Part model, mm, in its own coordinate system. A direction names the side the tool comes from. Round coordinates to 2 decimals unless told otherwise and drop trailing zeros. Write each loop counter-clockwise with the first axis right and the second up, starting at its lowest first coordinate (ties: lowest second). Pieces come first, ordered by that corner, then holes.
1) Saw through at D-D on x = -7.5. Write the cut outline in (y, z).
2) Flat gauge pins, fed straight in: pin 1 (14 mm diameter, centred on x = 0, y = 0, fed in from +Z); pin 2 (3 mm diameter, centred on x = 2, y = -10.5, fed in from -Z); pin 3 (4.5 mm diameter, centred on x = -18.415, z = 25.4, fed in from -Y); pin 4 (14 mm diameter, centred on x = -17.5, z = 38, fed in from +Y). Where does each tip first touch, or does it go through?
3) Which spindle directions (+Z, -Z, +X, -X, +Y, -Y) get a long thin tool onto all of the face, cutting with end or side? Do faces 1 (the flat face through (-1, -25.4, 25)), 2 (the flat face through (-1, -22.098, 27)). Say none if no direction does.
4) Saw through at A-A on z = 25.4. Write the cut outline in (x, y), and give its area (3 significant figures).
5) Pull direction Z, two halves, no side cores. Call faces 3 (the flat face through (-1, 7, 3.302)), 4 (the cylindrical face through (-16.01, -23.77, 28.02)), 5 (the flat face through (36.83, -23, 14)): +Z half, -Z half, draft (parallel to the pull), parting line (faces both ways), or undercut.
6) Saw through at B-B on y = 0. Write the cut outline in (x, z), and give its area (3 significant figures).
7) Saw through at C-C on x = 0. Write the cut outline in (y, z).
8) Drill centre lines: L1, parallel to X at y = -23.9, z = 25.4; L2, parallel to Y at x = 0, z = 1; L3, parallel to Y at x = -17.5, z = 14. Where is each one in solid material? Low to high.
```python
from build123d import *

# Parameters (mm, degrees)
SKETCH1_W           = 73.66
SKETCH1_H           = 50.8
BOSS_EXTRUDE2_DEPTH = 3.302
SKETCH4_W           = 73.66
SKETCH4_H           = 3.302
BOSS_EXTRUDE3_DEPTH = 47.498
SKETCH5_R           = 5.461
CUT_EXTRUDE2_DEPTH  = 68.692310494
SKETCH8_R           = 3.556
CUT_EXTRUDE3_DEPTH  = 81.732452583


with BuildPart() as part:
    # Sketch1 → Boss-Extrude2 (new body)
    with BuildSketch(Plane.XY):
        Rectangle(SKETCH1_W, SKETCH1_H)
    extrude(amount=BOSS_EXTRUDE2_DEPTH)

    # Sketch4 → Boss-Extrude3 (add)
    with BuildSketch(Plane.XY.offset(3.302)):
        with Locations((0, -23.749)):
            Rectangle(SKETCH4_W, SKETCH4_H)
    extrude(amount=BOSS_EXTRUDE3_DEPTH)

    # Sketch5 → Cut-Extrude2 (cut, through all)
    with BuildSketch(Plane(origin=(0, 0, 0), x_dir=(-1, 0, 0), z_dir=(0, 0, -1))):
        Circle(SKETCH5_R)
    extrude(amount=-CUT_EXTRUDE2_DEPTH, mode=Mode.SUBTRACT)

    # Sketch8 → Cut-Extrude3 (cut, through all)
    with BuildSketch(Plane.XZ.offset(25.4)):
        with Locations(Location((-18.415, 25.4, 0), (0, 0, 270))):
            Circle(SKETCH8_R)
        with Locations(Location((18.415, 25.4, 0), (0, 0, 270))):
            Circle(SKETCH8_R)
    extrude(amount=-CUT_EXTRUDE3_DEPTH, mode=Mode.SUBTRACT)


solid = part.part
```
Completed:
1. outline: (-25.4, 0) - (25.4, 0) - (25.4, 3.3) - (-22.1, 3.3) - (-22.1, 50.8) - (-25.4, 50.8) - close
2. pin 1: stops at z = 3.3
2. pin 2: stops at z = 0
2. pin 3: passes through
2. pin 4: stops at y = -22.1
3. face 1: +Z, -Z, +X, -X, -Y
3. face 2: +Z, +X, -X, +Y
4. outline: (-36.83, -25.4) - (-21.97, -25.4) - (-21.97, -22.1) - (-36.83, -22.1) - close; (-14.86, -25.4) - (14.86, -25.4) - (14.86, -22.1) - (-14.86, -22.1) - close; (21.97, -25.4) - (36.83, -25.4) - (36.83, -22.1) - (21.97, -22.1) - close
4. area: 196 mm2
5. face 3: +Z half
5. face 4: undercut
5. face 5: draft
6. outline: (-36.83, 0) - (-5.46, 0) - (-5.46, 3.3) - (-36.83, 3.3) - close; (5.46, 0) - (36.83, 0) - (36.83, 3.3) - (5.46, 3.3) - close
6. area: 207 mm2
7. outline: (-25.4, 0) - (-5.46, 0) - (-5.46, 3.3) - (-22.1, 3.3) - (-22.1, 50.8) - (-25.4, 50.8) - close; (5.46, 0) - (25.4, 0) - (25.4, 3.3) - (5.46, 3.3) - close
8. L1: x = -36.83 to -21.97, -14.86 to 14.86, 21.97 to 36.83
8. L2: y = -25.4 to -5.46, 5.46 to 25.4
8. L3: y = -25.4 to -22.1
